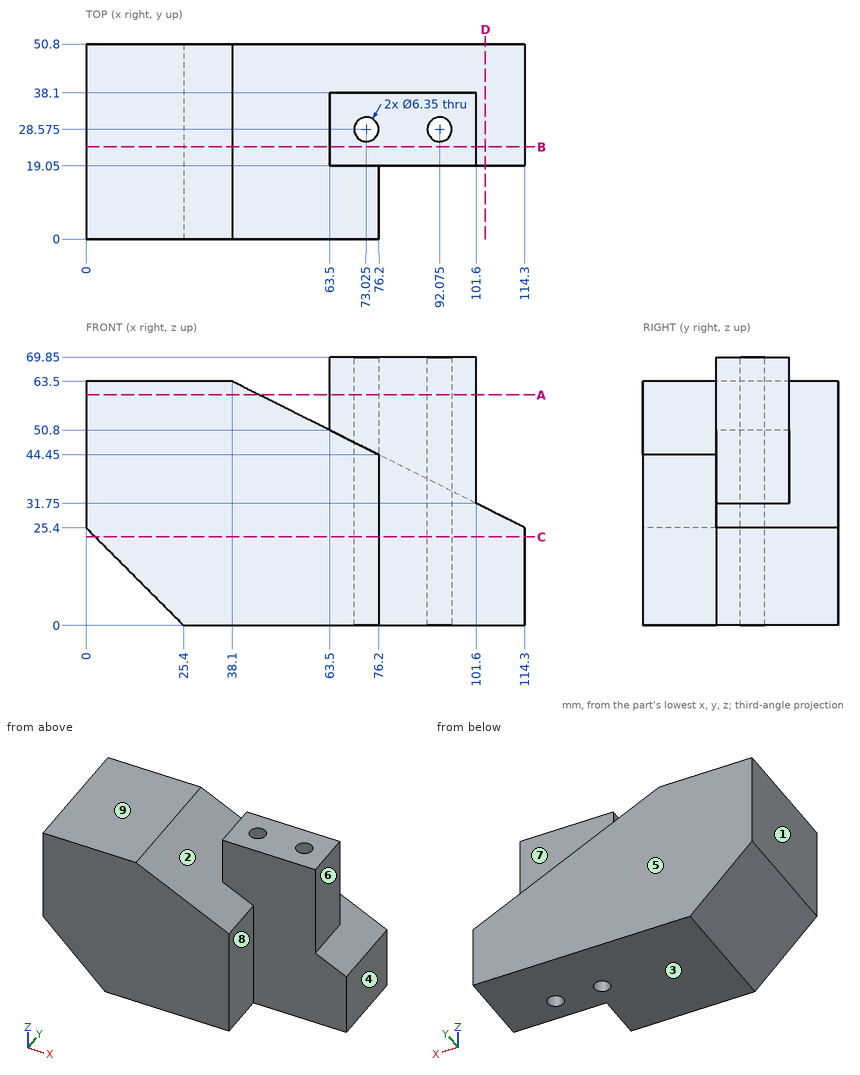
Design review of the part shown in the three views and the two pictorial views. Dimensions are in mm from the part's minimum x, y and z. A direction names the side the tool comes from. Give positions to 0.01 mm unless a question says otherwise; leave off trailing zeros. Write each loop counter-clockwise with the first axis right and the second up, starting at its lowest first coordinate (ties: lowest second). Pieces come first, ordered by that corner, then holes. Notation, with made-up numbers: M 0.5,62 L 18.5,62 A10 cw 18.5,79 Z; hole C 78.5,-32.75 d2. An arc over 180 degrees is marked long. Answer in a Markdown table with one row per item.
Item 1: Add section D-D on x = 104. Give the boundary of the cut face in (y, z), plus the area to 3 significant figures.
Check sheet entries:
| item | result |
|---|---|
| outline | M 19.05,0 L 50.8,0 L 50.8,30.55 L 19.05,30.55 Z |
| area | 970 mm2 |
Item 2: Add section B-B on y = 24. Give the boundary of the cut face in (x, z).
Check sheet entries:
| item | result |
|---|---|
| outline | M 0,25.4 L 25.4,0 L 114.3,0 L 114.3,25.4 L 101.6,31.75 L 101.6,69.85 L 63.5,69.85 L 63.5,50.8 L 38.1,63.5 L 0,63.5 Z |
Item 3: Tool access review of the marked faces 5, 6, 7, 8 and 9: name each direction out of +Z, -Z, +X, -X, +Y, -Y from which nothing blocks a thin tool from reaching the whole face with its end or side.
Check sheet entries:
| item | result |
|---|---|
| face 5 | +Z, -Z, +X, -X, +Y |
| face 6 | +Z, +X, +Y, -Y |
| face 7 | +Z, +X, +Y |
| face 8 | +Z, -Z, +X, -Y |
| face 9 | +Z, -X, +Y, -Y |
Item 4: Add section C-C on z = 23. Give the boundary of the cut face in (x, y) (3 decimals).
Check sheet entries:
| item | result |
|---|---|
| outline | M 2.4,0 L 76.2,0 L 76.2,19.05 L 114.3,19.05 L 114.3,50.8 L 2.4,50.8 Z; hole C 73.025,28.575 d6.35; hole C 92.075,28.575 d6.35 |
Item 5: For P1, Ø8, axis at x = 97, z = 48, coming from the -Y side; P2, Ø10, axis at y = 30.5, z = 29, coming from the -X side; P3, Ø1, axis at x = 45, y = 21, coming from the +Z side; P4, Ø9.5, axis at y = 9.5, z = 25.5, coming from the +X side, all flat-tipped, find the tip position at first contact; note any pin that passes through.
Check sheet entries:
| item | result |
|---|---|
| P1 | y = 19.05 |
| P2 | x = 0 |
| P3 | z = 60.3 |
| P4 | x = 76.2 |
Item 6: Add section A-A on z = 60. Give the boundary of the cut face in (x, y) (3 decimals), plus the area to 3 significant figures.
Check sheet entries:
| item | result |
|---|---|
| outline | M 0,0 L 45.1,0 L 45.1,50.8 L 0,50.8 Z; M 63.5,19.05 L 101.6,19.05 L 101.6,38.1 L 63.5,38.1 Z; hole C 73.025,28.575 d6.35; hole C 92.075,28.575 d6.35 |
| area | 2,950 mm2 |
Item 7: Draft analysis for pull direction X (two halves, no side actions). For the marked faces 1, 2, 3 and 4, state which applies: +X half, -X half, draft (parallel to the pull), parting line (faces both ways), or undercut.
Check sheet entries:
| item | result |
|---|---|
| face 1 | -X half |
| face 2 | undercut |
| face 3 | draft |
| face 4 | +X half |
Item 8: For line 1 along X through (y, z) = (30, 13.5); line 2 along X through (y, z) = (38, 64); line 3 along X through (y, z) = (27.5, 25.5), list the stretches that pass through material, from the lowest coordinate up.
Check sheet entries:
| item | result |
|---|---|
| line 1 | 11.9 to 70.19, 75.86 to 89.24, 94.91 to 114.3 |
| line 2 | 63.5 to 101.6 |
| line 3 | 0 to 70.04, 76.01 to 89.09, 95.06 to 114.1 |
